Here's how the part is built. I have some questions about the finished solid (model axes, mm). A direction names the side the tool comes from. Round coordinates to 2 decimals unless told otherwise and drop trailing zeros. Order: outer loops, then holes, each group sorted by start corner. A loop starts at its lowest first (then second) coordinate and runs counter-clockwise, first axis right, second up.
Autodesk Inventor part; units mm, degrees
ref_plane "YZ Plane" through (0, 0, 0) normal (1, 0, 0) x (0, 1, 0)
ref_plane "XZ Plane" through (0, 0, 0) normal (0, 1, 0) x (-1, 0, 0)
ref_plane "XY Plane" through (0, 0, 0) normal (0, 0, 1) x (1, 0, 0)
sketch "Sketch1" plane through (0, 0, 0) normal (0, 0, 1) x (1, 0, 0)
  line L0 (131.4017, -33.1581) -> (234.4053, -26.2304) construction
  line L1 (375.2105, -13.3271) -> (477.233, -67.9218) construction
  line L2 (380.4679, -2.1311) -> (480.5131, -62.4845)
  line L3 (480.5131, -62.4845) -> (473.953, -73.359)
  line L4 (369.9531, -24.5231) -> (473.953, -73.359)
  line L5 (380.4679, -2.1311) -> (369.9531, -24.5231) construction
  line L6 (128.7595, -60.7752) -> (134.1036, -4.9164) construction
  line L7 (128.7595, -60.7752) -> (-5.3656, -32.0813)
  circle A0 centre (-0.0519, -7.2434) radius 25.4
  line L8 (134.1036, -4.9164) -> (4.3231, 17.777)
  line L9 (131.4017, -33.1581) -> (-0.0519, -7.2434) construction
  line L10 (265.3565, -22.0515) -> (375.2105, -13.3271) construction
  line L11 (134.1036, -4.9164) -> (380.4679, -2.1311)
  line L12 (128.7595, -60.7752) -> (369.9531, -24.5231)
  circle A1 centre (471.6268, -64.9218) radius 3.175
  circle A2 centre (-0.0519, -7.2434) radius 3.175
  point P0 (0, 0)
  dimension "d4" = 148
  dimension "d5" = 50.8
  dimension "d6" = 24.7379
  dimension "d7" = 165
  dimension "d8" = 4.7
  dimension "d9" = 3.2
  dimension "d10" = 137.16
  dimension "d11" = 246.38
  dimension "d12" = 116.84
  dimension "d13" = 12.7
  dimension "d14" = 6.35
  dimension "d15" = 6.35
  dimension "d16" = 6.35
extrude "Extrusion1" add sketch "Sketch1" along normal mid plane 20.32 contours L2 L3 L4 L12 L7 A0 L8 L11
extrude "Extrusion2" add sketch "Sketch1" along normal mid plane 38.1 contours A0
properties part number "forearm"
1. If we section it at C-C, the plane y = 4: Write out the boundary of the cut face in (x, z).
Evaluation:
outline: (-22.83, -19.05) - (22.72, -19.05) - (22.72, -10.16) - (83.11, -10.16) - (83.11, 10.16) - (22.72, 10.16) - (22.72, 19.05) - (-22.83, 19.05) - close
2. I'm going to push flat-ended pins straight in: P1, Ø5, axis at y = -18.5, z = -2.5, coming from the -X side; P2, Ø10, axis at x = 318.5, y = -20, coming from the +Z side; P3, Ø3, axis at x = 287, z = 8.5, coming from the -Y side; P4, Ø7.5, axis at x = -0.05, y = -7.24, coming from the +Z side. Where does each tip first touch, or does it pass through?
Evaluation:
P1: stops at x = -23.89
P2: stops at z = 10.16
P3: stops at y = -37.22
P4: stops at z = 19.05
3. If we section it at B-B, the plane y = -47: Write out the boundary of the cut face in (x, z).
Evaluation:
outline: (64.37, -10.16) - (220.41, -10.16) - (220.41, 10.16) - (64.37, 10.16) - close; (417.82, -10.16) - (454.85, -10.16) - (454.85, 10.16) - (417.82, 10.16) - close
4. On a 3-axis mill with a long thin cutter (end or side, diameter ignored), from which of +Z, -Z, +X, -X, +Y, -Y can I reach the whole of each face in a straight line? I mean faces 1 (the flat face through (0, -13, 19.05)), 2 (the flat face through (247.7, -42.9, -0.1)), 3 (the cylindrical face through (-20.21, 8.21, -0.27)). Say none if no direction works.
Evaluation:
face 1: +Z, +X, -X, +Y, -Y
face 2: +Z, -Z, -Y
face 3: none
5. I need wall thicknesses on probe 1 along Z at (x, y) = (334.5, -7); probe 2 along X at (y, z) = (-9, -11); probe 3 along X at (y, z) = (-18, -2). Which ranges of each line are inside material? Lowest first, please.
Evaluation:
probe 1: z = -10.16 to 10.16
probe 2: x = -25.39 to -2.7, 2.59 to 25.29
probe 3: x = -23.06 to 406.77
6. If we section it at A-A, the plane z = -3: State how many separate pieces and enclosed holes the cut face has, and give its area (3 significant figures).
Evaluation:
separate pieces: 1
enclosed holes: 2
area: 19,600 mm2
7. If we section it at D-D, the plane x = 257: Write out the boundary of the cut face in (y, z).
Evaluation:
outline: (-41.5, -10.16) - (-3.53, -10.16) - (-3.53, 10.16) - (-41.5, 10.16) - close
